Verification items for the finished model (mm, model axes). A direction names the side the tool comes from. Give positions to 0.01 mm unless a question says otherwise; leave off trailing zeros. Write each loop counter-clockwise with the first axis right and the second up, starting at its lowest first coordinate (ties: lowest second). Pieces come first, ordered by that corner, then holes.
from build123d import *

# Parameters (mm, degrees)
SKETCH_1_W          = 20
SKETCH_1_H          = 10
EXTRUDE_1_DEPTH     = 5
CHAMFER_1_SIZE      = 1
CUT_EXTRUDE_1_DEPTH = 1


with BuildPart() as part:
    # 草图1 → 凸台-拉伸1 (new body)
    with BuildSketch(Plane.XY):
        Rectangle(SKETCH_1_W, SKETCH_1_H)
    extrude(amount=EXTRUDE_1_DEPTH)

    # 倒角1
    chamfer_1_edges = [part.edges().sort_by_distance(p)[0] for p in [
        (-10, 0, 5),
        (0, -5, 5),
        (10, 0, 5),
        (0, 5, 5),
    ]]
    chamfer(chamfer_1_edges, length=CHAMFER_1_SIZE)

    # 草图2 → 切除-拉伸1 (cut)
    with BuildSketch(Plane.XY.offset(5)):
        Polygon((-5.266489436, -2.668957232), (-5.510172516, -2.120670303), (-8.075856157, -3.260974143), (-7.832173078, -3.809261072), align=None)
        Polygon((-5.266489436, 2.668957232), (-7.832173078, 3.809261072), (-8.075856157, 3.260974143), (-5.510172516, 2.120670303), align=None)
        Polygon((5.266489436, 2.668957232), (5.510172516, 2.120670303), (8.075856157, 3.260974143), (7.832173078, 3.809261072), align=None)
        Polygon((5.266489436, -2.668957232), (7.832173078, -3.809261072), (8.075856157, -3.260974143), (5.510172516, -2.120670303), align=None)
    extrude(amount=-CUT_EXTRUDE_1_DEPTH, mode=Mode.SUBTRACT)


solid = part.part
Item 1: Scan lines: line 1 along Y through (x, z) = (6, 4.6); line 2 along Y through (x, z) = (-1.25, 4.25); line 3 along X through (y, z) = (-2, 4.1). Record each from-to range of solid material in increasing order.
Answer key:
line 1: y = -4.4 to -2.99, -2.34 to 2.34, 2.99 to 4.4
line 2: y = -4.75 to 4.75
line 3: x = -9.9 to 9.9
Item 2: Sectioned sample at C-C on y = -3. Record the cut outline in (x, z), then the cut area to 3 significant figures.
Answer key:
outline: (-10, 0) - (10, 0) - (10, 4) - (9, 5) - (7.49, 5) - (7.49, 4) - (6.01, 4) - (6.01, 5) - (-6.01, 5) - (-6.01, 4) - (-7.49, 4) - (-7.49, 5) - (-9, 5) - (-10, 4) - close
area: 96.0 mm2
Item 3: Release check for a two-part mould opening along X. For faces 3 (the face through (-10, 0, 2)), 4 (the face through (-6.57, -3.25, 4.51)), 5 (the face through (10, 0, 2)), 6 (the face through (-0.1, -4.5, 4.5)) record: released by +X, released by -X, zero draft, split by the parting line, or undercut.
Answer key:
face 3: released by -X
face 4: undercut
face 5: released by +X
face 6: zero draft
Item 4: Sectioned sample at A-A on z = 4.7. Record the cut outline in (x, y), then the cut area to 3 significant figures.
Answer key:
outline: (-9.3, -4.3) - (9.3, -4.3) - (9.3, 4.3) - (-9.3, 4.3) - close; hole (-8.08, -3.26) - (-7.83, -3.81) - (-5.27, -2.67) - (-5.51, -2.12) - close; hole (-8.08, 3.26) - (-5.51, 2.12) - (-5.27, 2.67) - (-7.83, 3.81) - close; hole (5.27, -2.67) - (7.83, -3.81) - (8.08, -3.26) - (5.51, -2.12) - close; hole (5.27, 2.67) - (5.51, 2.12) - (8.08, 3.26) - (7.83, 3.81) - close
area: 153 mm2
Item 5: Sectioned sample at B-B on x = -5. Record the cut outline in (y, z), then the cut area to 3 significant figures.
Answer key:
outline: (-5, 0) - (5, 0) - (5, 4) - (4, 5) - (-4, 5) - (-5, 4) - close
area: 49.0 mm2
Item 6: Sectioned sample at D-D on x = 7. Record the cut outline in (y, z).
Answer key:
outline: (-5, 0) - (5, 0) - (5, 4) - (4, 5) - (3.44, 5) - (3.44, 4) - (2.78, 4) - (2.78, 5) - (-2.78, 5) - (-2.78, 4) - (-3.44, 4) - (-3.44, 5) - (-4, 5) - (-5, 4) - close
Item 7: Set-up check for faces 1 (the face through (-9.5, -0.1, 4.5)), 2 (the face through (6.57, 3.25, 4.51)): record each of +Z, -Z, +X, -X, +Y, -Y from which the full face is reachable in a straight line by a thin tool's end or side.
Answer key:
face 1: +Z, -X, +Y, -Y
face 2: +Z
